Geometry check sheet. Reference: the model listing, model coordinates, mm. Round coordinates to 2 decimals unless told otherwise and drop trailing zeros. Write each loop counter-clockwise with the first axis right and the second up, starting at its lowest first coordinate (ties: lowest second). Pieces come first, ordered by that corner, then holes.
Item 1: Cross-section at B-B (x = 13.75). Enter the section's corners in (y, z) (3 decimals).
Item 2: Depth check by flat-ended pin: P1, Ø1.5, axis at y = 7.5, z = 115.5, coming from the +X side (3 decimals); P2, Ø10, axis at x = 12, y = 3, coming from the -Z side; P3, Ø4, axis at x = 5.5, y = 9, coming from the +Z side; P4, Ø14, axis at x = 11.5, z = 403, coming from the +Y side. Enter the tip coordinate at first touch or a pass-through.
Item 3: Scan lines: probe 1 along X at (y, z) = (8.5, 617) (3 decimals); probe 2 along X at (y, z) = (5, 383). Record each from-to range of solid material in increasing order.
Item 4: Cross-section at A-A (z = 689). Enter the section's corners in (x, y) (3 decimals), then the cut area to 3 significant figures.
Item 5: Cross-section at C-C (y = 18.5). Enter the section's corners in (x, z) (3 decimals).
Autodesk Inventor part; units mm, degrees
ref_plane "Start Plane" through (0, 0, 0) normal (0, 0, 1) x (1, 0, 0)
ref_plane "End Plane" through (0, 0, 750) normal (0, 0, 1) x (1, 0, 0)
ref_plane "Work Plane4" through (0, 12.7, 750) normal (0.7071, 0, 0.7071) x (0.7071, 0, -0.7071)
ref_plane "Start Plane" through (0, 0, 0) normal (0, 0, 1) x (1, 0, 0)
ref_plane "End Plane" through (0, 0, 750) normal (0, 0, 1) x (1, 0, 0)
sketch "Sketch" plane through (0, 0, 0) normal (0, 0, 1) x (1, 0, 0)
  line L0 (25.4, 0) -> (0, 0)
  line L1 (0, 0) -> (0, 25.4)
  line L2 (0, 25.4) -> (1.651, 25.4)
  line L3 (3.175, 23.876) -> (3.175, 6.477)
  line L4 (6.477, 3.175) -> (23.876, 3.175)
  line L5 (25.4, 1.651) -> (25.4, 0)
  line L6 (0, -11.0414) -> (0, 31.5385) construction
  line L7 (-11.0414, 0) -> (31.5385, 0) construction
  arc A0 (3.175, 6.477) -> (6.477, 3.175) centre (6.477, 6.477) ccw
  arc A1 (3.175, 23.876) -> (1.651, 25.4) centre (1.651, 23.876) ccw
  arc A2 (25.4, 1.651) -> (23.876, 3.175) centre (23.876, 1.651) ccw
  line L8 (0, 40.0545) -> (0, -19.5574) construction
  line L9 (-19.5574, 0) -> (40.0545, 0) construction
  point P0 (3.175, 25.4)
  point P1 (3.175, 3.175)
  point P2 (25.4, 3.175)
  dimension "d0" = 25.4
  dimension "d1" = 25.4
  dimension "d2" = 3.175
  dimension "d3" = 3.175
  dimension "d10" = 0
  dimension "d11" = 0
  dimension "d14" = 3.302
  dimension "d15" = 1.524
extrude "Body" add sketch "Sketch" along normal up to surface (750 mm away) from surface at 0
sketch "Sketch3" plane through (0, 0, 0) normal (0, 0, 1) x (1, 0, 0)
  line L0 (0, 0) -> (10, 0)
ref_plane "Work Plane3" through (0, 0, 0) normal (0, -1, 0) x (1, 0, 0)
ref_plane "Work Plane4" through (0, 12.7, 750) normal (0.7071, 0, 0.7071) x (0.7071, 0, -0.7071)
split "Split1" plane through (0, 12.7, 750) removes the side toward (0.7071, 0, 0.7071)
ref_plane "Work Plane5" through (0, 12.7, 0) normal (0.7071, 0, -0.7071) x (-0.7071, 0, -0.7071)
split "Split2" plane through (0, 12.7, 0) removes the side toward (0.7071, 0, -0.7071)
sketch "Sketch4" plane through (0, 0, 0) normal (0, -1, 0) x (1, 0, 0)
  line L0 (-2, 0) -> (12, 0)
  line L1 (-2, 750) -> (12, 750)
  dimension "d17" = 750
equation "\"d0\" = G_H"
equation "\"d1\" = G_H"
equation "\"d2\" = G_T"
equation "\"d3\" = G_T"
equation "\"d14\" = G_IR"
equation "\"d15\" = G_ER"
equation "\"d4\" = G_L"
equation "\"G_H\" = 25.4"
equation "\"G_T\" = 3.175"
equation "\"G_ER\" = 1.524"
equation "\"G_IR\" = 3.302"
equation "\"G_L\" = d17"
equation "\"ex\" = 0"
equation "\"G_OFFSET_START\" = 0"
equation "\"G_OFFSET_END\" = 0"
equation "\"d13\" = G_OFFSET_END + B_L"
equation "\"B_L\" = 750"
properties part number "AISC - L 1 x 1 x 1/8 - 29.528" material "Steel, Mild"
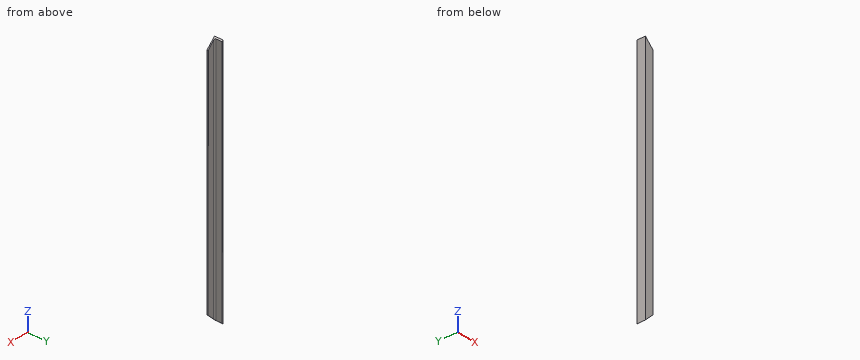
Resolved:
1. outline: (0, 13.75) - (3.175, 13.75) - (3.175, 736.25) - (0, 736.25) - close
2. P1: stops at x = 3.175
2. P2: stops at z = 7
2. P3: passes through
2. P4: stops at y = 3.83
3. probe 1: x = 0 to 3.175
3. probe 2: x = 0 to 3.52
4. outline: (0, 0) - (25.4, 0) - (25.4, 1.651) arc R1.524 ccw to (23.876, 3.175) - (6.477, 3.175) arc R3.302 cw to (3.175, 6.477) - (3.175, 23.876) arc R1.524 ccw to (1.651, 25.4) - (0, 25.4) - close
4. area: 153 mm2
5. outline: (0, 0) - (3.175, 3.175) - (3.175, 746.825) - (0, 750) - close
